from build123d import *

# Parameters (mm, degrees)
BOSS_EXTRUDE1_DEPTH = 50.8
SKETCH2_W           = 30.48
SKETCH2_H           = 50.8
BOSS_EXTRUDE2_DEPTH = 12.7
FILLET1_R           = 3.175
CHAMFER1_SIZE       = 6.35
FILLET2_R           = 6.35
FILLET3_R           = 6.35


with BuildPart() as part:
    # Sketch1 → Boss-Extrude1 (new body)
    with BuildSketch(Plane.XY):
        with BuildLine():
            Line((-36.801773982, 137.346090308), (-53.055841449, 198.007095926))
            Line((-53.055841449, 198.007095926), (-57.15, 198.007095926))
            Line((-57.15, 198.007095926), (-57.15, 96.407095926))
            Line((-57.15, 96.407095926), (57.15, 96.407095926))
            Line((57.15, 96.407095926), (57.15, 198.007095926))
            Line((57.15, 198.007095926), (53.055841449, 198.007095926))
            Line((53.055841449, 198.007095926), (36.801773982, 137.346090308))
            ThreePointArc((36.801773982, 137.346090308), (0, 109.107095926), (-36.801773982, 137.346090308))
        make_face()
    extrude(amount=BOSS_EXTRUDE1_DEPTH)

    # Sketch2 → Boss-Extrude2 (add)
    # profile 1 of 2: a face of its own
    with BuildSketch(Plane.XZ.offset(-96.407095926)):
        with Locations((-72.39, 25.4)):
            Rectangle(SKETCH2_W, SKETCH2_H)
        with BuildLine():
            Line((-77.47, 16.129), (-67.31, 16.129))
            ThreePointArc((-67.31, 16.129), (-63.881, 12.7), (-67.31, 9.271))
            Line((-67.31, 9.271), (-77.47, 9.271))
            ThreePointArc((-77.47, 9.271), (-80.899, 12.7), (-77.47, 16.129))
        make_face(mode=Mode.SUBTRACT)
        with BuildLine():
            Line((-77.47, 34.671), (-67.31, 34.671))
            ThreePointArc((-67.31, 34.671), (-63.881, 38.1), (-67.31, 41.529))
            Line((-67.31, 41.529), (-77.47, 41.529))
            ThreePointArc((-77.47, 41.529), (-80.899, 38.1), (-77.47, 34.671))
        make_face(mode=Mode.SUBTRACT)
    # profile 2 of 2: a face of its own
    with BuildSketch(Plane.XZ.offset(-96.407095926)):
        with Locations((72.39, 25.4)):
            Rectangle(SKETCH2_W, SKETCH2_H)
        with BuildLine():
            Line((77.47, 34.671), (67.31, 34.671))
            ThreePointArc((67.31, 34.671), (63.881, 38.1), (67.31, 41.529))
            Line((67.31, 41.529), (77.47, 41.529))
            ThreePointArc((77.47, 41.529), (80.899, 38.1), (77.47, 34.671))
        make_face(mode=Mode.SUBTRACT)
        with BuildLine():
            Line((77.47, 16.129), (67.31, 16.129))
            ThreePointArc((67.31, 16.129), (63.881, 12.7), (67.31, 9.271))
            Line((67.31, 9.271), (77.47, 9.271))
            ThreePointArc((77.47, 9.271), (80.899, 12.7), (77.47, 16.129))
        make_face(mode=Mode.SUBTRACT)
    extrude(amount=-BOSS_EXTRUDE2_DEPTH)

    # Fillet1
    fillet1_edges = [part.edges().sort_by_distance(p)[0] for p in [
        (-57.15, 109.107095926, 25.4),
        (57.15, 109.107095926, 25.4),
    ]]
    fillet(fillet1_edges, radius=FILLET1_R)

    # Chamfer1
    chamfer1_edges = [part.edges().sort_by_distance(p)[0] for p in [
        (-87.63, 102.757095926, 0),
        (-87.63, 102.757095926, 50.8),
        (87.63, 102.757095926, 0),
        (87.63, 102.757095926, 50.8),
    ]]
    chamfer(chamfer1_edges, length=CHAMFER1_SIZE)

    # Fillet2
    fillet2_edges = [part.edges().sort_by_distance(p)[0] for p in [
        (87.63, 102.757095926, 6.35),
        (87.63, 102.757095926, 44.45),
        (-87.63, 102.757095926, 44.45),
        (-87.63, 102.757095926, 6.35),
    ]]
    fillet(fillet2_edges, radius=FILLET2_R)

    # Fillet3
    # the kernel refuses this fillet: 6.35 mm, written as the material it takes off along each edge
    with BuildSketch(Plane(origin=(53.055841449, 198.007095926, -12.053098402), x_dir=(-0.2588190451025212, -0.9659258262890681, 0), z_dir=(0, 0, 1))) as fillet3_piece_1:
        with BuildLine():
            CenterArc((4.821239361, 6.35), FILLET3_R, 202.161584325, 67.838415675)
            Line((-1.059646207, 3.954653481), (-1.177263918, 3.906746551))
            ThreePointArc((-1.177263918, 3.906746551), (-0.652495683, 1.944456722), (-0.12267258, -0.032870019))
            Line((-0.12267258, -0.032870019), (0, -0.127))
            Line((0, -0.127), (4.821239361, -0.127))
            Line((4.821239361, -0.127), (4.821239361, 0))
        make_face()
    extrude(amount=74.906196803, mode=Mode.SUBTRACT)
    with BuildSketch(Plane(origin=(-53.055841449, 198.007095926, -12.053098402), x_dir=(-1, 0, 0), z_dir=(0, 0, 1))) as fillet3_piece_2:
        with BuildLine():
            CenterArc((4.885800429, 6.30046055), FILLET3_R, 195, 67.838415675)
            Line((-1.247828568, 4.656959613), (-1.370501147, 4.624089594))
            Line((-1.370501147, 4.624089594), (-0.12267258, -0.032870019))
            Line((-0.12267258, -0.032870019), (0, -0.127))
            ThreePointArc((0, -0.127), (2.047079275, -0.127), (4.078325713, -0.126009211))
            Line((4.078325713, -0.126009211), (4.094158551, 0))
        make_face()
    extrude(amount=74.906196803, mode=Mode.SUBTRACT)


solid = part.part
Can you work these out from the model? Positions are in its coordinate system, mm. A direction names the side the tool comes from. Coordinates: 2 decimals unless noted, no trailing zeros. Write each loop counter-clockwise with the first axis right and the second up, starting at its lowest first coordinate (ties: lowest second). Pieces come first, ordered by that corner, then holes. Notation, with made-up numbers: (22.25, -35.75) - (33.25, -35.75) arc R13 ccw to (33.25, -14.75) - close; hole circle Ø8 at (70.25, 69). An arc over 180 degrees is marked (long way). Return JSON: item names as keys, results as strings. Group by question number.
Item 1: We'd pull the mould along X, two halves only. Please class faces 6 (the face through (72, 103, 34.671)), 7 (the face through (87.133, 102.846, 44.282)), 8 (the face through (-87.63, 103, 25)), 9 (the face through (74, 109.107, 26)): pulls with the +X half, pulls with the -X half, needs draft (parallel to the pull), parting line crosses it, or undercut.
Item 2: If we section it at D-D (x = -44.5): Write out the boundary of the cut face in (y, z), then the cut area to 3 significant figures.
Item 3: Which directions (+Z, -Z, +X, -X, +Y, -Y) give clear straight access to the entire face, cutting with the end or side of a thin tool? Please do faces 1 (the face through (57.15, 155, 25)), 2 (the face through (-83.49, 102.67, 48.59)), 3 (the face through (-74, 109.107, 26)), 4 (the face through (-44.2, 164.96, 25.04)), 5 (the face through (-63.88, 102.67, 12.78)).
Item 4: If we section it at A-A (z = 38.1): Write out the boundary of the cut face in (x, y) (3 decimals), then the cut area to 3 significant figures.
Item 5: If we section it at C-C (y = 130.5): Write out the boundary of the cut face in (x, z), then the cut area to 3 significant figures.
Item 6: I'm going to push flat-ended pins straight in: pin 1 Ø12 at (x, y) = (-40, 173) entering from -Z; pin 2 Ø2 at (y, z) = (150.5, 32) entering from +X; pin 3 Ø12 at (x, z) = (-56, 7) entering from +Y; pin 4 Ø8 at (x, z) = (69, 18) entering from +Y. Where does each tip first touch, or does it pass through?
Item 7: If we section it at B-B (y = 171.5): Write out the boundary of the cut face in (x, z).
Item 8: Please list where these lines run through material, in increasing order: probe 1 along Y at (x, z) = (-61, 6.5); probe 2 along X at (y, z) = (126, 40.5); probe 3 along X at (y, z) = (192.5, 48).
Return value:
{
 "1": {"face 6": "undercut", "face 7": "pulls with the +X half", "face 8": "pulls with the -X half", "face 9": "needs draft"},
 "2": {"outline": "(96.41, 0) - (166.08, 0) - (166.08, 50.8) - (96.41, 50.8) - close", "area": "3,540 mm^2"},
 "3": {"face 1": "+Z, -Z, +X, +Y", "face 2": "+Z, -X, +Y, -Y", "face 3": "+Z, -Z, -X, +Y", "face 4": "+Z, -Z, +Y", "face 5": "+Y, -Y"},
 "4": {"outline": "(-87.63, 96.407) - (-80.899, 96.407) - (-80.899, 109.107) - (-87.63, 109.107) - close; (-63.881, 96.407) - (63.881, 96.407) - (63.881, 109.107) - (60.325, 109.107) arc R3.175 cw to (57.15, 112.282) - (57.15, 198.007) arc R6.35 ccw to (51.808, 193.35) - (36.802, 137.346) arc R38.1 cw to (-36.802, 137.346) - (-51.808, 193.35) arc R6.35 ccw to (-57.15, 198.007) - (-57.15, 112.282) arc R3.175 cw to (-60.325, 109.107) - (-63.881, 109.107) - close; (80.899, 96.407) - (87.63, 96.407) - (87.63, 109.107) - (80.899, 109.107) - close", "area": "4,960 mm^2"},
 "5": {"outline": "(-57.15, 0) - (-34.24, 0) - (-34.24, 50.8) - (-57.15, 50.8) - close; (34.24, 0) - (57.15, 0) - (57.15, 50.8) - (34.24, 50.8) - close", "area": "2,330 mm^2"},
 "6": {"pin 1": "passes through", "pin 2": "stops at x = 57.15", "pin 3": "stops at y = 198.01", "pin 4": "stops at y = 109.11"},
 "7": {"outline": "(-57.15, 0) - (-45.95, 0) - (-45.95, 50.8) - (-57.15, 50.8) - close; (45.95, 0) - (57.15, 0) - (57.15, 50.8) - (45.95, 50.8) - close"},
 "8": {"probe 1": "y = 96.41 to 109.11", "probe 2": "x = -57.15 to -31.65, 31.65 to 57.15", "probe 3": "x = -57.15 to -51.58, 51.58 to 57.15"}
}
